from build123d import *

# Parameters (mm, degrees)
SKETCH2_R                = 32
BOSS_EXTRUDE1_DEPTH      = 3
M3_CLEARANCE_HOLE1_D     = 3.4
M3_CLEARANCE_HOLE1_DEPTH = 4
M3_CLEARANCE_HOLE1_TIP   = 1.021463052


with BuildPart() as part:
    # Sketch1 → Revolve1 (revolve)
    with BuildSketch(Plane.XY, mode=Mode.PRIVATE) as revolve1_sk:
        Polygon((-26.5, -7.3), (-34, -4.3), (-34, 0), (0, 0), (0, -7.3), align=None)
    revolve(revolve1_sk.sketch.rotate(Axis((0, -7.3, 0), (0, 1, 0)), 270), axis=Axis((0, -7.3, 0), (0, 1, 0)))

    # Sketch2 → Boss-Extrude1 (add)
    with BuildSketch(Plane(origin=(0, 0, 0), x_dir=(1, 0, 0), z_dir=(0, 1, 0))):
        with Locations(Location((0, 0, 0), (0, 0, 270))):
            Circle(SKETCH2_R)
    extrude(amount=BOSS_EXTRUDE1_DEPTH)

    # M3 Clearance Hole1
    with Locations(Plane(origin=(0, -7.3, 0), x_dir=(-1, 0, 0), z_dir=(0, -1, 0))):
        with Locations((15.556349186, -15.556349186), (15.556349186, 15.556349186), (-15.556349186, 15.556349186), (-15.556349186, -15.556349186)):
            Hole(M3_CLEARANCE_HOLE1_D / 2, depth=M3_CLEARANCE_HOLE1_DEPTH)
            with Locations((0, 0, -(M3_CLEARANCE_HOLE1_DEPTH + M3_CLEARANCE_HOLE1_TIP / 2))):  # 118° drill point
                Cone(0, M3_CLEARANCE_HOLE1_D / 2, M3_CLEARANCE_HOLE1_TIP, mode=Mode.SUBTRACT)


solid = part.part
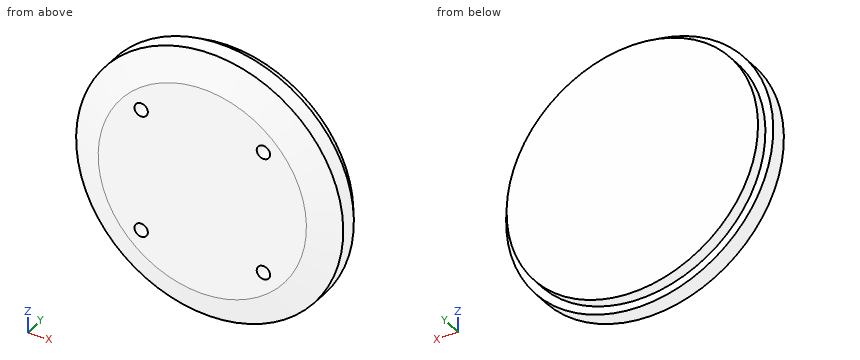
Source: CAD feature listing. Evaluate the final solid. Frame: model axes, mm. Coordinates: 2 decimals unless noted, no trailing zeros. Loops run counter-clockwise (first coordinate to the right, second up) from the corner with the lowest first, then second, coordinate; pieces in that order, holes last. Notation, with made-up numbers: (66, -17) - (119, -17) arc R19 cw to (119, -10) - close; hole circle Ø11 at (26.5, 30.25). An arc over 180 degrees is marked (long way). One line per item, written item: value. Start each with the question number.
1. Section B-B (z = 0). Return the cut outline in (x, y), and give its area (3 significant figures).
2. Contact query for flat-ended pins moving along their axis: P1, Ø6, axis at x = -24, y = -5, coming from the -Z side; P2, Ø2, axis at x = -16.5, z = 26, coming from the -Y side; P3, Ø5, axis at y = -4, z = -16.5, coming from the +X side; P4, Ø3, axis at x = -14, z = 15.5, coming from the -Y side. Output: stop coordinate, or through.
3. Section A-A (x = 0). Return the cut outline in (y, z).
4. Section D-D (y = -1). Return the cut outline in (x, z).
5. Section C-C (y = -5.5). Return the cut outline in (x, z).
6. Ray query, L1, parallel to Z at x = -27.5, y = -3.75; L2, parallel to Z at x = 6, y = -2.75; L3, parallel to X at y = -2.75, z = 29. Return the intervals inside material, ascending.
Verdict:
1. outline: (-34, -4.3) - (-26.5, -7.3) - (26.5, -7.3) - (34, -4.3) - (34, 0) - (32, 0) - (32, 3) - (-32, 3) - (-32, 0) - (-34, 0) - close
1. area: 666 mm2
2. P1: stops at z = -26.67
2. P2: stops at y = -5.98
2. P3: stops at x = 30.98
2. P4: stops at y = -7.3
3. outline: (-7.3, -26.5) - (-4.3, -34) - (0, -34) - (0, -32) - (3, -32) - (3, 32) - (0, 32) - (0, 34) - (-4.3, 34) - (-7.3, 26.5) - close
4. outline: circle Ø68 at (0, 0)
5. outline: circle Ø62 at (0, 0); hole circle Ø3.4 at (-15.56, -15.56); hole circle Ø3.4 at (-15.56, 15.56); hole circle Ø3.4 at (15.56, -15.56); hole circle Ø3.4 at (15.56, 15.56)
6. L1: z = -19.99 to 19.99
6. L2: z = -33.47 to 33.47
6. L3: x = -17.75 to 17.75
